Autodesk Inventor part; units mm, degrees
ref_plane "Start Plane" through (0, 0, 25.4) normal (0, 0, 1) x (1, 0, 0)
ref_plane "End Plane" through (0, 0, 381) normal (0, 0, 1) x (1, 0, 0)
ref_plane "Work Plane4" through (304.8, -25.4, 381) normal (0, 0, 1) x (1, 0, 0)
ref_plane "Start Plane" through (0, 0, 25.4) normal (0, 0, 1) x (1, 0, 0)
ref_plane "End Plane" through (0, 0, 381) normal (0, 0, 1) x (1, 0, 0)
sketch "Sketch" plane through (0, 0, 0) normal (0, 0, 1) x (1, 0, 0)
  line L0 (-25.4, -25.4) -> (-25.4, 25.4)
  line L1 (-12.7, 38.1) -> (12.7, 38.1)
  line L2 (25.4, 25.4) -> (25.4, -25.4)
  line L3 (12.7, -38.1) -> (-12.7, -38.1)
  arc A0 (-25.4, -25.4) -> (-12.7, -38.1) centre (-12.7, -25.4) ccw
  arc A1 (-12.7, 38.1) -> (-25.4, 25.4) centre (-12.7, 25.4) ccw
  arc A2 (25.4, 25.4) -> (12.7, 38.1) centre (12.7, 25.4) ccw
  arc A3 (12.7, -38.1) -> (25.4, -25.4) centre (12.7, -25.4) ccw
  arc A4 (-12.7, 31.75) -> (-19.05, 25.4) centre (-12.7, 25.4) ccw
  line L4 (-12.7, 31.75) -> (12.7, 31.75)
  arc A5 (19.05, 25.4) -> (12.7, 31.75) centre (12.7, 25.4) ccw
  line L5 (19.05, 25.4) -> (19.05, -25.4)
  arc A6 (12.7, -31.75) -> (19.05, -25.4) centre (12.7, -25.4) ccw
  line L6 (12.7, -31.75) -> (-12.7, -31.75)
  arc A7 (-19.05, -25.4) -> (-12.7, -31.75) centre (-12.7, -25.4) ccw
  line L7 (-19.05, -25.4) -> (-19.05, 25.4)
  line L8 (0, 57.0224) -> (0, -57.0224) construction
  line L9 (-39.2424, 0) -> (39.2424, 0) construction
  dimension "d10" = 76.2
  dimension "d11" = 50.8
  dimension "d12" = 6.35
  dimension "d15" = 38.1
  dimension "d16" = 25.4
  dimension "d17" = 12.7
extrude "Body" add sketch "Sketch" along normal up to surface (355.6 mm away) from surface at 25.4
sketch "Sketch3" plane through (0, 0, 0) normal (0, 0, 1) x (1, 0, 0)
  line L0 (0, 0) -> (10, 0)
ref_plane "Work Plane3" through (0, 0, 0) normal (0, -1, 0) x (1, 0, 0)
ref_plane "Work Plane4" through (304.8, -25.4, 381) normal (0, 0, 1) x (1, 0, 0)
split "Split1" plane through (304.8, -25.4, 381) removes the side toward (0, 0, 1)
ref_plane "Work Plane5" through (-609.6, -25.4, 25.4) normal (0, 0, -1) x (-1, 0, 0)
split "Split2" plane through (-609.6, -25.4, 25.4) removes the side toward (0, 0, -1)
ref_plane "Work Plane6" through (-20.32, -25.4, 15.24) normal (0.8, 0, -0.6) x (-0.6, 0, -0.8)
split "Split3" plane through (-20.32, -25.4, 15.24) removes the side toward (0.8, 0, -0.6)
sketch "Sketch4" plane through (0, 0, 0) normal (0, -1, 0) x (1, 0, 0)
  line L0 (-2, 25.4) -> (12, 25.4)
  line L1 (-2, 381) -> (12, 381)
  dimension "d19" = 355.6
equation "\"d10\" = G_H"
equation "\"d11\" = G_W"
equation "\"d12\" = G_T"
equation "\"d15\" = 0.5 * d10"
equation "\"d16\" = 0.5 * d11"
equation "\"d17\" = G_IR"
equation "\"d3\" = G_L"
equation "\"G_W\" = 50.8"
equation "\"G_H\" = 76.2"
equation "\"G_T\" = 6.35"
equation "\"G_IR\" = 12.7"
equation "\"G_L\" = d19"
equation "\"G_OFFSET_START\" = -25.4"
equation "\"G_OFFSET_END\" = -25.4"
equation "\"d13\" = -G_OFFSET_START"
equation "\"d14\" = G_OFFSET_END + B_L"
equation "\"B_L\" = 406.4"
properties part number "AISC - 3 x 2 x 1/4 - 14" material "Steel, Mild"
Input: part model. Units: mm. Frame: model coordinates. A direction names the side the tool comes from. Round coordinates to 2 decimals unless told otherwise and drop trailing zeros. Order: outer loops, then holes, each group sorted by start corner. A loop starts at its lowest first (then second) coordinate and runs counter-clockwise, first axis right, second up. Notation, with made-up numbers: (73, 74.25) - (96, 74.25) arc R26 ccw to (96, 111.25) - close; hole circle Ø2 at (-33, 25). An arc over 180 degrees is marked (long way). Answer in a Markdown table with one row per item.
Item 1: Section query C-C (z = 282.5). Return the cut outline in (x, y).
Model answer:
| item | result |
|---|---|
| outline | (-25.4, -25.4) arc R12.7 ccw to (-12.7, -38.1) - (12.7, -38.1) arc R12.7 ccw to (25.4, -25.4) - (25.4, 25.4) arc R12.7 ccw to (12.7, 38.1) - (-12.7, 38.1) arc R12.7 ccw to (-25.4, 25.4) - close; hole (-19.05, -25.4) arc R6.35 ccw to (-12.7, -31.75) - (12.7, -31.75) arc R6.35 ccw to (19.05, -25.4) - (19.05, 25.4) arc R6.35 ccw to (12.7, 31.75) - (-12.7, 31.75) arc R6.35 ccw to (-19.05, 25.4) - close |
Item 2: Section query A-A (y = -8). Return the cut outline in (x, z).
Model answer:
| item | result |
|---|---|
| outline | (-25.4, 25.4) - (-19.05, 25.4) - (-19.05, 381) - (-25.4, 381) - close; (19.05, 67.73) - (25.4, 76.2) - (25.4, 381) - (19.05, 381) - close |
Item 3: Line query: line 1 (X direction, y = -12, z = 263); line 2 (Y direction, x = 8.5, z = 129); line 3 (Y direction, x = 13, z = 333.5). Output: solid intervals per line, ascending.
Model answer:
| item | result |
|---|---|
| line 1 | x = -25.4 to -19.05, 19.05 to 25.4 |
| line 2 | y = -38.1 to -31.75, 31.75 to 38.1 |
| line 3 | y = -38.1 to -31.74, 31.74 to 38.1 |
Item 4: Pin query (flat end, axial travel): pin 1 (12 mm diameter, centred on x = 13, y = -28, fed in from -Z). Return the tip coordinate at first contact, or that it passes through.
Model answer:
| item | result |
|---|---|
| pin 1 | stops at z = 53.42 |
Item 5: Section query B-B (x = -7). Return the cut outline in (y, z).
Model answer:
| item | result |
|---|---|
| outline | (-38.1, 33) - (-31.75, 33) - (-31.75, 381) - (-38.1, 381) - close; (31.75, 33) - (38.1, 33) - (38.1, 381) - (31.75, 381) - close |
Item 6: Reachability of faces 1 (the flat face through (19.05, 0, 222)), 2 (the cylindrical face through (-21.78, 34.28, 200.71)) from +Z, -Z, +X, -X, +Y, -Y: full face, straight path, thin tool, end or side. Return the list, or none.
Model answer:
| item | result |
|---|---|
| face 1 | +Z, -Z |
| face 2 | +Z, -Z, -X, +Y |
Item 7: Mould query, pull axis X, two halves, no side actions, for faces 3 (the cylindrical face through (17.24, -29.84, 217.88)), 4 (the cylindrical face through (17.14, 29.94, 217.88)), 5 (the flat face through (25.4, 0, 226)), 6 (the flat face through (0, -38.1, 201)). Classes: released by +X, released by -X, zero draft, split by the parting line, or undercut.
Model answer:
| item | result |
|---|---|
| face 3 | undercut |
| face 4 | undercut |
| face 5 | released by +X |
| face 6 | zero draft |
